The listing builds one solid part. Answer for the finished solid, in the listing's coordinates (mm). A direction names the side the tool comes from. Round coordinates to 2 decimals unless told otherwise and drop trailing zeros. Order: outer loops, then holes, each group sorted by start corner. A loop starts at its lowest first (then second) coordinate and runs counter-clockwise, first axis right, second up. Notation, with made-up numbers: (-19.5, 38.25) - (6.5, 38.25) arc R31 ccw to (6.5, 67.25) - close; hole circle Ø10 at (19.5, 32). An arc over 180 degrees is marked (long way). Use CSV: the item, a comma, the result in double quotes. Start each with the question number.
Item 1: Find section C-C, the plane x = 12. Give the vertices of the cut face in (y, z).
Item 2: Determine the mould class of faces 4 (the flat face through (38, 2, -93.79)), 5 (the flat face through (21, 2, 90.488)), 6 (the flat face through (7.826, 2, -92)), 7 (the flat face through (41.402, 2, -26)) for opening direction X: +X half, -X half, draft (parallel to the pull), parting line (faces both ways), or undercut.
Item 3: Find section A-A, the plane x = -14.5. Give the vertices of the cut face in (y, z), plus the area to 3 significant figures.
Item 4: Straight lines are drawn through the part: line 1 along Z through (x, y) = (-2.5, 2.4); line 2 along X through (y, z) = (2.85, 14) (3 decimals); line 3 along Z through (x, y) = (-10, 2). For each, find the intervals that lie inside material, in ascending order. Write a range as [from, to].
Item 5: Flat-ended cylindrical pins translate along their axes: P1, Ø1.7, axis at y = 1.5, z = -54, coming from the -X side; P2, Ø1, axis at x = 23, y = 1, coming from the -Z side; P3, Ø1, axis at y = 1.5, z = 53, coming from the -X side. Find the tip coordinate at first contact, or state that the pin passes through.
Item 6: For faces 1 (the flat face through (-40, 2, -66.207)), 2 (the flat face through (21, 2, -90.488)), 3 (the flat face through (-19.685, 2, 1)), determine the directions among +Z, -Z, +X, -X, +Y, -Y from which every point of the face is accessible in a straight line to the end or side of a thin tool.
Item 7: Find section B-B, the plane z = 6.5. Give the vertices of the cut face in (x, y) (3 decimals), plus the area to 3 significant figures.
Autodesk Inventor part; units mm, degrees
ref_plane "YZ Plane" through (0, 0, 0) normal (1, 0, 0) x (0, 1, 0)
ref_plane "XZ Plane" through (0, 0, 0) normal (0, 1, 0) x (-1, 0, 0)
ref_plane "XY Plane" through (0, 0, 0) normal (0, 0, 1) x (1, 0, 0)
sketch "Sketch1" plane through (0, 0, 0) normal (0, 1, 0) x (-1, 0, 0)
  line L0 (-38.1, 90.4875) -> (38.1, 90.4875) construction
  line L1 (38.1, 90.4875) -> (38.1, -90.4875) construction
  line L2 (38.1, -90.4875) -> (-38.1, -90.4875) construction
  line L3 (-38.1, -90.4875) -> (-38.1, 90.4875) construction
  line L4 (-38.1, 90.4875) -> (38.1, -90.4875) construction
  line L5 (38.1, 90.4875) -> (-38.1, -90.4875) construction
  line L6 (19.05, 77.7875) -> (0, 77.7875) construction
  line L7 (0, 77.7875) -> (0, -77.7875) construction
  line L8 (0, -77.7875) -> (19.05, -77.7875) construction
  line L9 (19.05, -77.7875) -> (19.05, 77.7875) construction
  line L10 (41.402, 93.7895) -> (-41.402, 93.7895)
  line L11 (-41.402, 93.7895) -> (-41.402, -93.7895)
  line L12 (-41.402, -93.7895) -> (41.402, -93.7895)
  line L13 (41.402, -93.7895) -> (41.402, 93.7895)
  line L14 (41.402, 93.7895) -> (-41.402, -93.7895) construction
  line L15 (-41.402, 93.7895) -> (41.402, -93.7895) construction
  line L16 (19.685, -78.4225) -> (-0.635, -78.4225)
  line L17 (-0.635, -78.4225) -> (-0.635, 78.4225)
  line L18 (-0.635, 78.4225) -> (19.685, 78.4225)
  line L19 (19.685, 78.4225) -> (19.685, -78.4225)
  point P0 (0, 0)
  point P1 (0, 0)
  point P2 (0, 0)
  point P3 (9.525, -78.4225)
  point P4 (9.525, -77.7875)
  point P5 (19.685, 0)
  point P6 (19.05, 0)
  dimension "d0" = 19.05
  dimension "d1" = 155.575
  dimension "d2" = 3.302
  dimension "d3" = 3.302
  dimension "d4" = 12.7
  dimension "d5" = 19.05
  dimension "d6" = 38.1
  dimension "d7" = 0.635
  dimension "d8" = 0.635
extrude "Extrusion1" add sketch "Sketch1" along normal blind 3.302
sketch "Sketch2" plane through (0, 0, 0) normal (0, 1, 0) x (-1, 0, 0)
  line L0 (-41.402, 93.7895) -> (-41.402, -93.7895)
  line L1 (-41.402, -93.7895) -> (41.402, -93.7895)
  line L2 (41.402, -93.7895) -> (41.402, 93.7895)
  line L3 (41.402, 93.7895) -> (-41.402, 93.7895)
  line L4 (33.576, -93.7895) -> (7.826, -93.7895)
  line L5 (7.826, -93.7895) -> (7.826, -90.4875)
  line L6 (7.826, -90.4875) -> (33.576, -90.4875)
  line L7 (33.576, -90.4875) -> (33.576, -93.7895)
  line L8 (-7.826, -93.7895) -> (-33.576, -93.7895)
  line L9 (-33.576, -93.7895) -> (-33.576, -90.4875)
  line L10 (-33.576, -90.4875) -> (-7.826, -90.4875)
  line L11 (-7.826, -90.4875) -> (-7.826, -93.7895)
  line L12 (0, -131.3053) -> (0, 131.3053)
  line L13 (-66.8528, 0) -> (66.8528, 0)
  line L14 (-41.402, -66.2073) -> (-38.1, -66.2073)
  line L15 (-38.1, -66.2073) -> (-38.1, -40.4572)
  line L16 (-38.1, -40.4572) -> (-41.402, -40.4572)
  line L17 (-41.402, -40.4572) -> (-41.402, -66.2073)
  line L18 (-41.402, -12.875) -> (-38.1, -12.875)
  line L19 (-38.1, -12.875) -> (-38.1, 12.875)
  line L20 (-38.1, 12.875) -> (-41.402, 12.875)
  line L21 (-41.402, 12.875) -> (-41.402, -12.875)
  line L22 (-41.402, 40.4572) -> (-38.1, 40.4572)
  line L23 (-38.1, 40.4572) -> (-38.1, 66.2073)
  line L24 (-38.1, 66.2073) -> (-41.402, 66.2073)
  line L25 (-41.402, 66.2073) -> (-41.402, 40.4572)
  line L26 (38.1, 50.3478) -> (36.5506, 50.3477)
  line L27 (36.5506, 50.3477) -> (36.5506, 56.3167)
  line L28 (36.5506, 56.3167) -> (38.1, 56.3167)
  line L29 (38.1, 56.3167) -> (38.1, 50.3478)
  point P0 (0, 0)
  point P1 (20.701, -90.4875)
  point P2 (-38.1, -53.3322)
  point P3 (36.5506, 53.3322)
  point P4 (-38.1, 53.3322)
  dimension "d11" = 25.75
  dimension "d13" = 3.302
  dimension "d14" = 41.402
  dimension "d15" = 20.701
  dimension "d19" = 3.302
  dimension "d24" = 40.4573
  dimension "d25" = 80.9145
  dimension "d33" = 1.5494
  dimension "d34" = 5.969
  dimension "d35" = 3.302
  dimension "d36" = 40.4573
extrude "Extrusion2" cut sketch "Sketch2" along normal blind 3.302 contours L24 L23 L22 L0 | L20 L19 L13 L0 | L19 L18 L0 L13 | L16 L15 L14 L0
extrude "Extrusion3" cut sketch "Sketch2" along normal blind 3.302 contours L1 L9 L10 L11 | L5 L6 L7 L1
mirror "Mirror1" about plane through (0, 0, 0) normal (1, 0, 0) of "Extrusion2"
mirror "Mirror2" about plane through (0, 0, 0) normal (0, 0, 1) of "Extrusion3"
extrude "Extrusion4" cut sketch "Sketch2" along normal blind 3.302 contours L26 L27 L28 L29
equation "\"d2\" = encThick"
equation "\"d3\" = encThick"
equation "\"d9\" = encThick"
equation "\"d13\" = encThick"
equation "\"d19\" = d13"
equation "\"d35\" = encThick"
equation "\"d26\" = encThick"
equation "\"d28\" = encThick"
equation "\"d37\" = encThick"
equation "\"encThick\" = 3.302"
equation "\"encTab\" = 25.4"
equation "\"antOffset\" = d36"
properties part number "Enclosure Top" material "Glass"
Worked out:
1,outline,"(0, -90.49) - (3.3, -90.49) - (3.3, 90.49) - (0, 90.49) - close"
2,face 4,"draft"
2,face 5,"undercut"
2,face 6,"undercut"
2,face 7,"+X half"
3,outline,"(0, -90.49) - (3.3, -90.49) - (3.3, -78.42) - (0, -78.42) - close; (0, 78.42) - (3.3, 78.42) - (3.3, 90.49) - (0, 90.49) - close"
3,area,"79.7 mm²"
4,line 1,"z = [-93.79, -78.42], [78.42, 93.79]"
4,line 2,"x = [-41.402, -19.685], [0.635, 41.402]"
4,line 3,"z = [-90.49, -78.42], [78.42, 90.49]"
5,P1,"stops at x = -38.1"
5,P2,"stops at z = -90.49"
5,P3,"stops at x = -36.55"
6,face 1,"-X, +Y, -Y"
6,face 2,"-Z, +Y, -Y"
6,face 3,"+Y, -Y"
7,outline,"(-38.1, 0) - (-19.685, 0) - (-19.685, 3.302) - (-38.1, 3.302) - close; (0.635, 0) - (38.1, 0) - (38.1, 3.302) - (0.635, 3.302) - close"
7,area,"185 mm²"
